The model under review builds one solid part; all positions refer to its coordinate system, in mm. Face numbers are marked on the shaded views. Round coordinates to 2 decimals unless told otherwise and drop trailing zeros. Order: outer loops, then holes, each group sorted by start corner. A loop starts at its lowest first (then second) coordinate and runs counter-clockwise, first axis right, second up. Notation, with made-up numbers: M 49.5,33 L 96.5,33 A29 cw 96.5,56 Z; hole C -17,82.5 d10. An arc over 180 degrees is marked long. One line per item, written item: value. Start each with the question number.
from build123d import *

# Parameters (mm, degrees)
F0_R     = 25.5
F1_DEPTH = 50
F0_R_2   = 11.625
F2_DEPTH = 9
F4_R     = 8
F5_DEPTH = 15
F8_D     = 3
F8_DEPTH = 8
F8_TIP   = 0.9012909285


with BuildPart() as f1:
    # F0 (on Top) → F1 (new body)
    with BuildSketch(Plane.XY):
        with BuildLine():
            Line((21.5, 26.5), (-21.5, 26.5))
            ThreePointArc((-21.5, 26.5), (-25.0355339059, 25.0355339059), (-26.5, 21.5))
            Line((-26.5, 21.5), (-26.5, -21.5))
            ThreePointArc((-26.5, -21.5), (-25.0355339059, -25.0355339059), (-21.5, -26.5))
            Line((-21.5, -26.5), (21.5, -26.5))
            ThreePointArc((21.5, -26.5), (25.0355339059, -25.0355339059), (26.5, -21.5))
            Line((26.5, -21.5), (26.5, 21.5))
            ThreePointArc((26.5, 21.5), (25.0355339059, 25.0355339059), (21.5, 26.5))
        make_face()
        Circle(F0_R, mode=Mode.SUBTRACT)
    extrude(amount=F1_DEPTH)

    # F0 (on Top) → F2 (join)
    with BuildSketch(Plane.XY):
        Circle(F0_R)
        Circle(F0_R_2, mode=Mode.SUBTRACT)
    extrude(amount=F2_DEPTH)

    # F4 (on offset) → F5 (cut)
    with BuildSketch(Plane.YZ.offset(26.5)):
        with Locations((13.5627460668, 24)):
            Circle(F4_R)
    extrude(amount=-F5_DEPTH, mode=Mode.SUBTRACT)

    # F8
    with Locations(Plane.XY.offset(50)):
        with Locations((-21.5, 21.5), (21.5, 21.5), (21.5, -21.5), (-21.5, -21.5)):
            Hole(F8_D / 2, depth=F8_DEPTH)
            with Locations((0, 0, -(F8_DEPTH + F8_TIP / 2))):  # 118° drill point
                Cone(0, F8_D / 2, F8_TIP, mode=Mode.SUBTRACT)


solid = f1.part
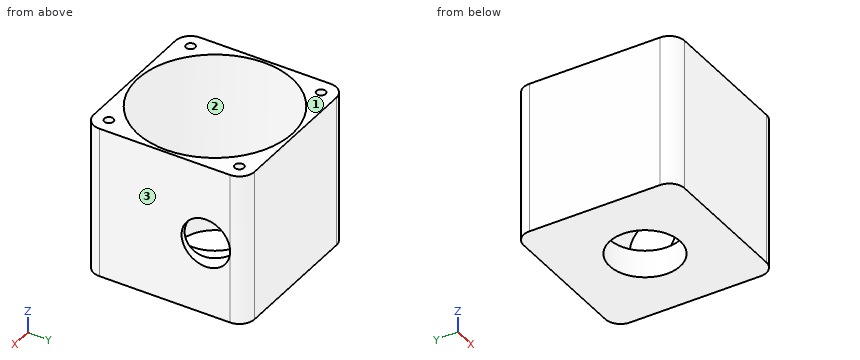
Item 1: The part is to be moulded in two halves that separate along X. For the marked faces 1, 2 and 3, say which applies: pulls with the +X half, pulls with the -X half, needs draft (parallel to the pull), parting line crosses it, or undercut.
Item 2: Consider section B-B, the plane y = 0. Give the boundary of the cut face in (x, z) (3 decimals).
Item 3: Clearance check with flat-ended pins moving along their axes: P1, Ø18.5, axis at x = 0, y = 0, coming from the -Z side; P2, Ø9.5, axis at y = 13.56, z = 24, coming from the +X side. State where each tip first meets the part, or that it passes through.
Item 4: Wall thickness on L1, parallel to Y at x = 0, z = 24; L2, parallel to X at y = -21.5, z = 46.5: over which ranges is each line inside the solid? List them lowest first.
Item 5: Consider section A-A, the plane z = 4.5. Give the boundary of the cut face in (x, y) (3 decimals).
Item 6: Consider section D-D, the plane y = 7. Give the boundary of the cut face in (x, z), then the cut area to 3 significant figures.
Computed:
1. face 1: needs draft
1. face 2: undercut
1. face 3: pulls with the +X half
2. outline: M -26.5,0 L -11.625,0 L -11.625,9 L -25.5,9 L -25.5,50 L -26.5,50 Z; M 11.625,0 L 26.5,0 L 26.5,50 L 25.5,50 L 25.5,9 L 11.625,9 Z
3. P1: passes through
3. P2: stops at x = -17.75
4. L1: y = -26.5 to -25.5, 25.5 to 26.5
4. L2: x = -26.5 to -23, -20 to -13.71, 13.71 to 20, 23 to 26.5
5. outline: M -26.5,-21.5 A5 ccw -21.5,-26.5 L 21.5,-26.5 A5 ccw 26.5,-21.5 L 26.5,21.5 A5 ccw 21.5,26.5 L -21.5,26.5 A5 ccw -26.5,21.5 Z; hole C 0,0 d23.25
6. outline: M -26.5,0 L -9.28,0 L -9.28,9 L -24.52,9 L -24.52,50 L -26.5,50 Z; M 9.28,0 L 26.5,0 L 26.5,19.43 L 24.52,19.43 L 24.52,9 L 9.28,9 Z; M 24.52,28.57 L 26.5,28.57 L 26.5,50 L 24.52,50 Z
6. area: 454 mm^2
